Geometry check sheet. Reference: the model listing, model coordinates, mm. A direction names the side the tool comes from. Give positions to 0.01 mm unless a question says otherwise; leave off trailing zeros. Write each loop counter-clockwise with the first axis right and the second up, starting at its lowest first coordinate (ties: lowest second). Pieces come first, ordered by that corner, then holes.
(1) Cross-section at D-D (x = -1.25). Count the separate pieces of the cut face and the enclosed holes in it, and give its area (3 significant figures).
(2) Depth check by flat-ended pin: P1, Ø3, axis at x = -2.5, y = -7, coming from the +Z side. Enter the tip coordinate at first touch or a pass-through.
(3) Cross-section at B-B (x = 0). Record the boundary of the cut face in (y, z), and give its area (3 significant figures).
(4) Thickness scan on line 1 along Y through (x, z) = (0, 2.05); line 2 along X through (y, z) = (0, 2.2); line 3 along Y through (x, z) = (-1, 1.25). Record the ranges inside material, lowest first.
(5) Cross-section at C-C (z = 6). Record the boundary of the cut face in (x, y), and give its area (3 significant figures).
(6) Mould release check, pull along Y, two halves, no side actions. Record for faces 1 (the cylindrical face through (-0.577, -1.439, 2.068)), 2 (the flat face through (0, -2, -0.2)), 3 (the cylindrical face through (0.1, -11.5, 5.2)): +Y half, -Y half, draft (parallel to the pull), parting line (faces both ways), or undercut.
(7) Tool access check on faces 4 (the cylindrical face through (-0.1, 4.5, 5.2)), 5 (the flat face through (0, -3, 4.2)). Record the directions out of +Z, -Z, +X, -X, +Y, -Y that give a thin tool (end or side, any length) a straight path to the whole face; none if there is none.
(8) Cross-section at A-A (z = 0.5). Record the boundary of the cut face in (x, y), and give its area (3 significant figures).
Autodesk Inventor part; units mm, degrees
ref_plane "YZ Plane" through (0, 0, 0) normal (1, 0, 0) x (0, 1, 0)
ref_plane "XZ Plane" through (0, 0, 0) normal (0, 1, 0) x (-1, 0, 0)
ref_plane "XY Plane" through (0, 0, 0) normal (0, 0, 1) x (1, 0, 0)
sketch "Skizze1" plane through (0, 0, 0) normal (0, 0, 1) x (1, 0, 0)
  circle A0 centre (0, 0) radius 2.7
  circle A1 centre (0, -7) radius 2.7
  dimension "d22" = 5.4
  dimension "d23" = 7
extrude "Extrusion1" add sketch "Skizze1" along normal blind 5.2
sketch "Skizze2" plane through (0, 0, 5.2) normal (0, 0, 1) x (1, 0, 0)
  arc A0 (-3, -7) -> (3, -7) centre (0, -7) ccw
  arc A1 (-3, -7) -> (3, -7) centre (0, -7) ccw
  line L0 (-3, 0) -> (-3, -7)
  arc A2 (3, 0) -> (-3, 0) centre (0, 0) ccw
  line L1 (3, -7) -> (3, 0)
  arc A3 (-3, -7) -> (3, -7) centre (0, -7) ccw
  line L2 (-3, 0) -> (-3, -7)
  arc A4 (-3, -7) -> (3, -7) centre (0, -7) ccw
  line L3 (3, -7) -> (3, 0)
  arc A5 (3, 0) -> (-3, 0) centre (0, 0) ccw
  line L4 (-3, 0) -> (-3, -7)
  line L5 (-3, 0) -> (-3, -7)
  arc A6 (-3, -7) -> (3, -7) centre (0, -7) ccw
  arc A7 (-3, -7) -> (3, -7) centre (0, -7) ccw
  line L6 (3, -7) -> (3, 0)
  line L7 (3, -7) -> (3, 0)
  arc A8 (3, 0) -> (-3, 0) centre (0, 0) ccw
  arc A9 (3, 0) -> (-3, 0) centre (0, 0) ccw
  line L8 (-4.5, 0) -> (-4.5, -7)
  arc A10 (-4.5, -7) -> (4.5, -7) centre (0, -7) ccw
  line L9 (4.5, -7) -> (4.5, 0)
  arc A11 (4.5, 0) -> (-4.5, 0) centre (0, 0) ccw
  dimension "d4" = 9
extrude "Extrusion2" add sketch "Skizze2" along normal blind 2 contours L0 A2 L1 A0 | A11 L9 A10 L8
sketch "Skizze3" plane through (0, 0, 7.2) normal (0, 0, 1) x (1, 0, 0)
  point P0 (0, 0)
  point P1 (0, 0)
  point P2 (0, -7)
  dimension "d7" = 7
hole "Bohrung1" at (0, 0, 7.2) at (0, -7, 7.2) direction (0, 0, -1) diameter 3.1 end through all
chamfer "Fasen1" distance 2.8 angle 45 2 edges at (0, 1.55, 7.2) (0, -5.45, 7.2)
sketch "Skizze5" plane through (0, 0, 5.2) normal (0, 0, -1) x (-1, 0, 0)
  circle A0 centre (0, -7) radius 2.7
  line L0 (4.5, 0) -> (4.5, -7)
  arc A1 (-4.5, -7) -> (4.5, -7) centre (0, -7) ccw
  line L1 (-4.5, -7) -> (-4.5, 0)
  arc A2 (4.5, 0) -> (-4.5, 0) centre (0, 0) ccw
  circle A3 centre (0, 0) radius 2.7
  circle A4 centre (0, -7) radius 2.35
  circle A5 centre (0, 0) radius 2.35
extrude "Extrusion4" add sketch "Skizze5" along normal blind 1 contours L0 A1 L1 A2
sketch "Skizze6" plane through (0, 0, 7.2) normal (0, 0, 1) x (1, 0, 0)
  arc A0 (-2.5831, -3.5) -> (2.5831, -3.5) centre (0, -7) ccw
  arc A1 (2.5831, -3.5) -> (-2.5831, -3.5) centre (0, 0) ccw
  arc A2 (-4.5, -7) -> (4.5, -7) centre (0, -7) ccw
  line L0 (-4.5, -7) -> (-4.5, 0)
  arc A3 (4.5, 0) -> (-4.5, 0) centre (0, 0) ccw
  line L1 (4.5, 0) -> (4.5, -7)
extrude "Extrusion5" cut sketch "Skizze6" against normal blind 1 contours A1 A0 | L0 A3 L1 A2
sketch "Skizze7" plane through (0, 0, 0) normal (0, 0, -1) x (-1, 0, 0)
  circle A0 centre (0, 0) radius 1.55
  circle A1 centre (0, 0) radius 2.7
  circle A2 centre (0, -7) radius 1.55
  circle A3 centre (0, -7) radius 2.7
extrude "Extrusion6" add sketch "Skizze7" along normal blind 0.2
properties part number "Stange halter"
Reply:
1. separate pieces: 3
1. enclosed holes: 0
1. area: 41.6 mm2
2. P1: stops at z = 6.2
3. outline: (-11.5, 4.2) - (-9.7, 4.2) - (-9.7, -0.2) - (-8.55, -0.2) - (-8.55, 4.4) - (-10.35, 6.2) - (-11.5, 6.2) - close; (-5.45, -0.2) - (-4.3, -0.2) - (-4.3, 4.2) - (-2.7, 4.2) - (-2.7, -0.2) - (-1.55, -0.2) - (-1.55, 4.4) - (-3.35, 6.2) - (-3.65, 6.2) - (-5.45, 4.4) - close; (1.55, -0.2) - (2.7, -0.2) - (2.7, 4.2) - (4.5, 4.2) - (4.5, 6.2) - (3.35, 6.2) - (1.55, 4.4) - close
3. area: 33.4 mm2
4. line 1: y = -9.7 to -8.55, -5.45 to -4.3, -2.7 to -1.55, 1.55 to 2.7
4. line 2: x = -2.7 to -1.55, 1.55 to 2.7
4. line 3: y = -9.51 to -8.18, -5.82 to -4.49, -2.51 to -1.18, 1.18 to 2.51
5. outline: (-4.5, -7) arc R4.5 ccw to (4.5, -7) - (4.5, 0) arc R4.5 ccw to (-4.5, 0) - close; hole circle Ø6.3 at (0, -7); hole circle Ø6.3 at (0, 0)
5. area: 64.3 mm2
6. face 1: undercut
6. face 2: draft
6. face 3: -Y half
7. face 4: +Z, -Z, +Y
7. face 5: -Z
8. outline: circle Ø5.4 at (0, -7); circle Ø5.4 at (0, 0); hole circle Ø3.1 at (0, -7); hole circle Ø3.1 at (0, 0)
8. area: 30.7 mm2
